Geometry: see drawing. Coordinates: mm, zero at the bounding-box minimum. A direction names the side the tool comes from. Give positions to 0.01 mm unless a question says otherwise; leave off trailing zeros. Write each loop counter-clockwise with the first axis right and the second up, starting at its lowest first coordinate (ties: lowest second). Pieces come first, ordered by that corner, then holes.
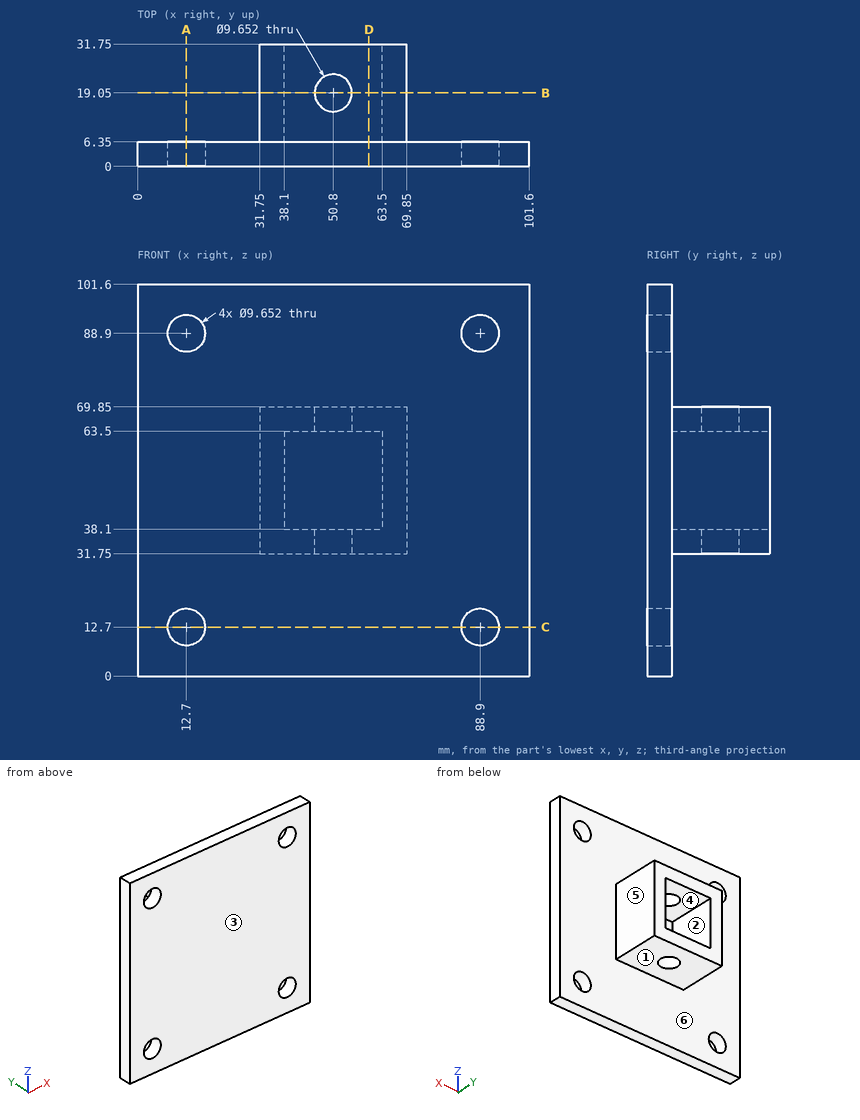
1. Section query A-A (x = 12.7). Return loops of the section in (y, z).
2. Line query: probe 1 along Z at (x, y) = (88.9, 4.5); probe 2 along X at (y, z) = (3, 88); probe 3 along Y at (x, z) = (50.8, 37.25). Output: solid intervals per line, ascending.
3. Pin query (flat end, axial travel): P1, Ø10, axis at x = 13.5, z = 53, coming from the +Y side; P2, Ø10, axis at y = 12, z = 28.5, coming from the -X side; P3, Ø12.5, axis at x = 48.5, y = 15.5, coming from the -Z side; P4, Ø11, axis at x = 12.7, z = 12.7, coming from the -Y side. Return the tip coordinate at first contact, or that it passes through.
4. Section query D-D (x = 60). Return loops of the section in (y, z).
5. Section query C-C (z = 12.7). Return loops of the section in (x, y).
6. Section query B-B (y = 19.05). Return loops of the section in (x, z), plus the area to 3 significant figures.
7. Pull-direction query (Z, two-part tool) for the marked faces 1, 2, 3 and 4; classes: pulls with the +Z half, pulls with the -Z half, needs draft (parallel to the pull), parting line crosses it, or undercut.
8. Access query for the marked faces 5 and 6. Directions: +Z, -Z, +X, -X, +Y, -Y. A direction counts if a zero-diameter tool reaches every point of the face in a straight line with its end or side. Return the directions, or none.
The answers:
1. outline: (0, 0) - (6.35, 0) - (6.35, 7.87) - (0, 7.87) - close; (0, 17.53) - (6.35, 17.53) - (6.35, 84.07) - (0, 84.07) - close; (0, 93.73) - (6.35, 93.73) - (6.35, 101.6) - (0, 101.6) - close
2. probe 1: z = 0 to 7.87, 17.53 to 84.07, 93.73 to 101.6
2. probe 2: x = 0 to 7.96, 17.44 to 84.16, 93.64 to 101.6
2. probe 3: y = 0 to 14.22, 23.88 to 31.75
3. P1: stops at y = 6.35
3. P2: stops at x = 31.75
3. P3: stops at z = 31.75
3. P4: stops at y = 0
4. outline: (0, 0) - (6.35, 0) - (6.35, 31.75) - (31.75, 31.75) - (31.75, 38.1) - (6.35, 38.1) - (6.35, 63.5) - (31.75, 63.5) - (31.75, 69.85) - (6.35, 69.85) - (6.35, 101.6) - (0, 101.6) - close
5. outline: (0, 0) - (7.87, 0) - (7.87, 6.35) - (0, 6.35) - close; (17.53, 0) - (84.07, 0) - (84.07, 6.35) - (17.53, 6.35) - close; (93.73, 0) - (101.6, 0) - (101.6, 6.35) - (93.73, 6.35) - close
6. outline: (31.75, 31.75) - (45.97, 31.75) - (45.97, 38.1) - (38.1, 38.1) - (38.1, 63.5) - (45.97, 63.5) - (45.97, 69.85) - (31.75, 69.85) - close; (55.63, 31.75) - (69.85, 31.75) - (69.85, 69.85) - (55.63, 69.85) - (55.63, 63.5) - (63.5, 63.5) - (63.5, 38.1) - (55.63, 38.1) - close
6. area: 684 mm2
7. face 1: pulls with the -Z half
7. face 2: undercut
7. face 3: needs draft
7. face 4: undercut
8. face 5: +Z, -Z, +X, +Y
8. face 6: +Y
